Can you work these out from the drawing? Everything is in mm from the part's minimum corner. Give positions to 0.01 mm unless a question says otherwise; leave off trailing zeros. Write each loop counter-clockwise with the first axis right and the second up, starting at its lowest first coordinate (ties: lowest second). Pieces come first, ordered by that corner, then holes. Notation, with made-up numbers: (-36, 49) -> (-31, 49) arc R26 ccw to (-31, 67) -> close; hole circle Ø11 at (5.5, 72.5). An arc over 180 degrees is marked (long way). Return JSON: item names as keys, results as strings.
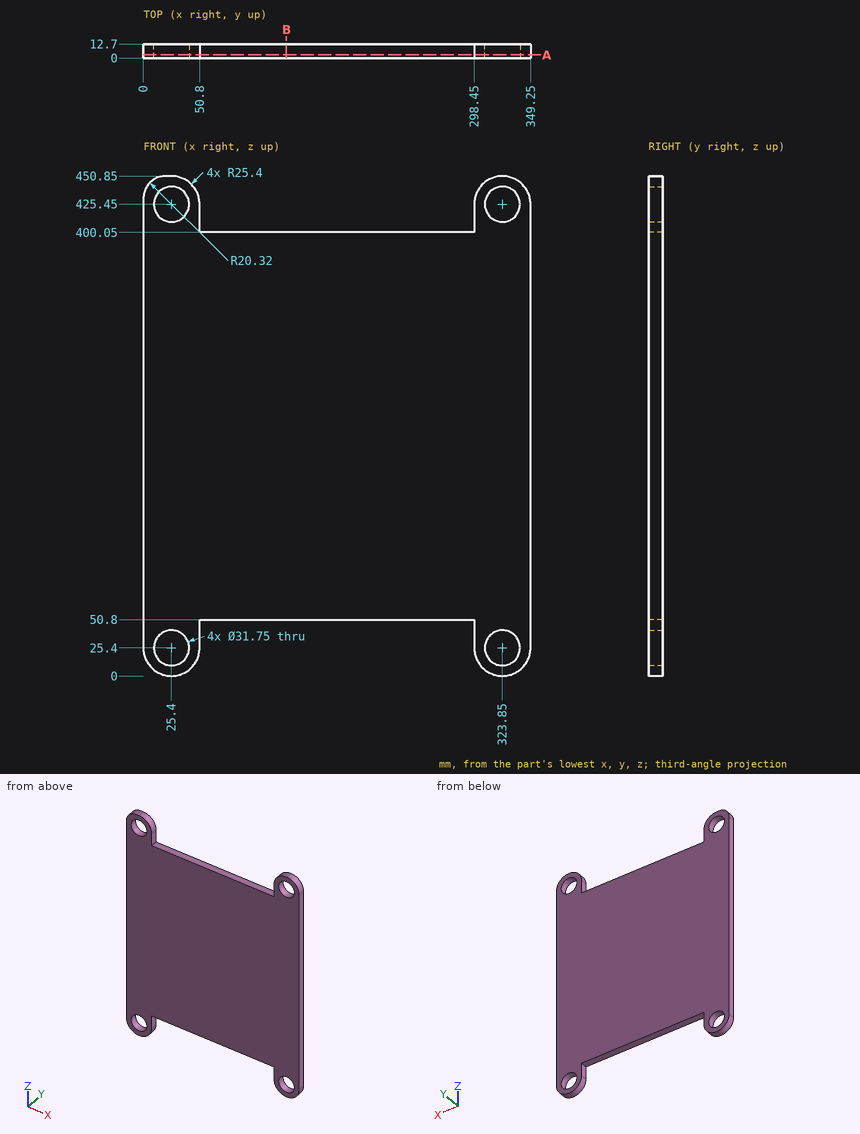
1. If I drill on line 1 (Z direction, x = 323.85, y = 9.75) (3 decimals); line 2 (X direction, y = 3.75, z = 405); line 3 (Z direction, x = 319, y = 0.5), over which ranges is the centre line in solid material (lowest first)? Write a range as [from, to].
Taken from the geometry:
{"line 1": "z = [0, 9.525], [41.275, 409.575], [441.325, 450.85]", "line 2": "x = [0, 50.8], [298.45, 349.25]", "line 3": "z = [0.47, 10.28], [40.52, 410.33], [440.57, 450.38]"}
2. Suppose I cut it at A-A, the plane y = 3. List the corners of the cut face in (x, z) for me (3 decimals).
Taken from the geometry:
{"outline": "(0, 25.4) arc R25.4 ccw to (25.4, 0) arc R25.4 ccw to (50.8, 25.4) -> (50.8, 50.8) -> (298.45, 50.8) -> (298.45, 25.4) arc R25.4 ccw to (323.85, 0) arc R25.4 ccw to (349.25, 25.4) -> (349.25, 425.45) arc R25.4 ccw to (323.85, 450.85) arc R25.4 ccw to (298.45, 425.45) -> (298.45, 400.05) -> (50.8, 400.05) -> (50.8, 425.45) arc R25.4 ccw to (25.4, 450.85) -> (20.32, 450.85) arc R20.32 ccw to (0, 430.53) -> close; hole circle Ø31.75 at (25.4, 25.4); hole circle Ø31.75 at (25.4, 425.45); hole circle Ø31.75 at (323.85, 25.4); hole circle Ø31.75 at (323.85, 425.45)"}
3. For pin 1 Ø4 at (x, y) = (284.5, 10.5) entering from +Z, with a flat end and sliding along its axis, tell me the tip position at first contact or that it passes through.
Taken from the geometry:
{"pin 1": "stops at z = 400.05"}
4. Suppose I cut it at B-B, the plane x = 129. List the corners of the cut face in (y, z) for me, and give its area (3 significant figures).
Taken from the geometry:
{"outline": "(0, 50.8) -> (12.7, 50.8) -> (12.7, 400.05) -> (0, 400.05) -> close", "area": "4,440 mm²"}
